Geometry: final body of the model. Coordinates: model frame, mm. A direction names the side the tool comes from. Round coordinates to 2 decimals unless told otherwise and drop trailing zeros. Loops run counter-clockwise (first coordinate to the right, second up) from the corner with the lowest first, then second, coordinate; pieces in that order, holes last. Notation, with made-up numbers: (34, 73.25) - (41, 73.25) arc R17 cw to (41, 102.25) - close; hole circle Ø8 at (-9, 3). An arc over 180 degrees is marked (long way). Answer as CSV lines item,"result".
from build123d import *

# Parameters (mm, degrees)
SKETCH001_R  = 4.1
POCKET_DEPTH = 25.001


with BuildPart() as part:
    # Sketch → Revolution (revolve)
    with BuildSketch(Plane.XZ):
        with BuildLine():
            Line((-17.5, 0), (-17.5, 25))
            Line((-17.5, 25), (-20.5, 25))
            Line((-20.5, 25), (-20.5, 21))
            Line((-20.5, 21), (-23.5, 21))
            Line((-23.5, 21), (-23.5, 25))
            Line((-23.5, 25), (-26.5, 25))
            Line((-26.5, 25), (-26.5, 20))
            ThreePointArc((-25, 18.5), (-25.43934, 19.56066), (-26.5, 20))
            Line((-25, 18.5), (-25, 6.5))
            ThreePointArc((-26.5, 5), (-25.43934, 5.43934), (-25, 6.5))
            Line((-26.5, 0), (-26.5, 5))
            Line((-23.5, 0), (-26.5, 0))
            Line((-23.5, 4), (-23.5, 0))
            Line((-20.5, 4), (-23.5, 4))
            Line((-20.5, 0), (-20.5, 4))
            Line((-17.5, 0), (-20.5, 0))
        make_face()
    revolve(axis=Axis((0, 0, 0), (0, 0, 1)))

    # Sketch001 (on Face1 of Revolution) → Pocket (cut, through all)
    with BuildSketch(Plane(origin=(0, 0, 0), x_dir=(1, 0, 0), z_dir=(0, 0, -1))):
        with Locations((20, 0)):
            Circle(SKETCH001_R)
        with Locations((-20, 0)):
            Circle(SKETCH001_R)
        with BuildLine():
            ThreePointArc((-20.070435, -20.480395), (-5.721449, -16.464083), (7.731739, -10.058157))
            Line((10.26, -14.371844), (7.731739, -10.058157))
            ThreePointArc((-19.14, -25.393062), (-3.96636, -21.145927), (10.26, -14.371844))
            Line((-20.070435, -20.480395), (-19.14, -25.393062))
        make_face()
    extrude(amount=-POCKET_DEPTH, mode=Mode.SUBTRACT)


solid = part.part
(1) Section B-B (z = 2). Output: boundary loops of the cut face in (x, y).
Findings below:
outline,"(-23.39, -2.31) arc R4.1 cw to (-23.39, 2.31) arc R23.5 cw to (-13.77, 19.04) arc R87 ccw to (-17.45, 19.94) arc R26.5 ccw (long way) to (-11.85, 23.7) arc R92 cw to (-7.32, 22.33) arc R23.5 cw to (23.39, 2.31) arc R4.1 cw to (23.39, -2.31) arc R23.5 cw to start; (-20.09, -4.1) arc R20.5 ccw to (20.09, -4.1) arc R4.1 cw to (17.24, -3.03) arc R17.5 cw to (-17.24, -3.03) arc R4.1 cw to start; (-20.09, 4.1) arc R4.1 cw to (-17.24, 3.03) arc R17.5 cw to (-5.82, 16.5) arc R87 ccw to (-9.95, 17.93) arc R20.5 ccw to start; (-2.04, 20.4) arc R92 cw to (10.26, 14.37) - (10.18, 14.23) arc R17.5 cw to (17.24, 3.03) arc R4.1 cw to (20.09, 4.1) arc R20.5 ccw to start"
(2) Pin query (flat end, axial travel): P1, Ø4, axis at x = -20.5, y = 18, coming from the -Z side; P2, Ø3, axis at x = -3.5, z = 10, coming from the +Y side; P3, Ø5, axis at x = 6.5, z = 21.5, coming from the +Y side; P4, Ø2, axis at x = 20.5, y = 8, coming from the +Z side. Return the tip coordinate at first contact, or that it passes through.
Findings below:
P1,"z = 0"
P2,"y = 24.92"
P3,"y = 26.2"
P4,"z = 21"
(3) Access query for faces 5 (the face through (-0.342, -17.497, 12.675)), 6 (the face through (-20.305, 11.83, 23.028)), 7 (the face through (11, 18, 4)). Directions: +Z, -Z, +X, -X, +Y, -Y. A direction counts if a zero-diameter tool reaches every point of the face in a straight line with its end or side. Return the directions, or none.
Findings below:
face 5,"+Z, -Z"
face 6,"+Z"
face 7,"-Z"
(4) Section A-A (y = 0). Output: boundary loops of the cut face in (x, z), and give its area (3 significant figures).
Findings below:
outline,"(-26.5, 0) - (-24.1, 0) - (-24.1, 25) - (-26.5, 25) - (-26.5, 20) arc R1.5 cw to (-25, 18.5) - (-25, 6.5) arc R1.5 cw to (-26.5, 5) - close; (24.1, 0) - (26.5, 0) - (26.5, 5) arc R1.5 cw to (25, 6.5) - (25, 18.5) arc R1.5 cw to (26.5, 20) - (26.5, 25) - (24.1, 25) - close"
area,"76.9 mm2"
(5) Draft query along Y for faces 1 (the face through (13.83, -22.605, 22.465)), 2 (the face through (12, 13, 25)), 3 (the face through (-0.393, -20.496, 22.972)), 4 (the face through (-0.645, 19.827, 12.325)). Return one class per face: pulls with the +Y half, pulls with the -Y half, needs draft (parallel to the pull), parting line crosses it, or undercut.
Findings below:
face 1,"parting line crosses it"
face 2,"needs draft"
face 3,"undercut"
face 4,"undercut"
(6) Material intervals for line 1 along X through (y, z) = (0, 15.5); line 2 along Y through (x, z) = (3, 22.5); line 3 along Y through (x, z) = (-20, 17.75), sorted ascending.
Findings below:
line 1,"-25 to -24.1, 24.1 to 25"
line 2,"-26.33 to -23.31, -20.28 to -17.24, 18.2 to 20.28, 23.31 to 26.33"
line 3,"-15 to -4.1, 4.1 to 15"
(7) Section D-D (x = -8). Give the number of separate pieces and of enclosed holes in the cut face, and give its area (3 significant figures).
Findings below:
separate pieces,"3"
enclosed holes,"0"
area,"282 mm2"
